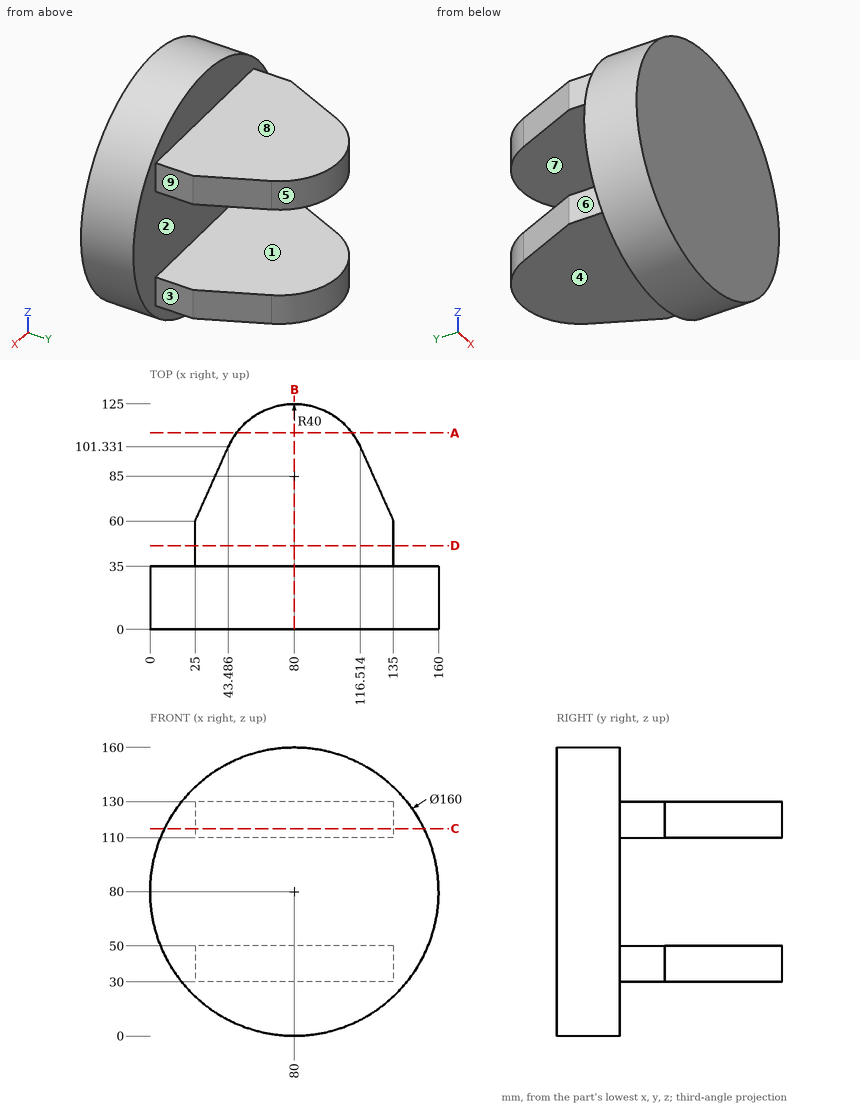
Geometry: see drawing. Coordinates: mm, zero at the bounding-box minimum. A direction names the side the tool comes from. Give positions to 0.01 mm unless a question says otherwise; leave off trailing zeros. Loops run counter-clockwise (first coordinate to the right, second up) from the corner with the lowest first, then second, coordinate; pieces in that order, holes last. Notation, with made-up numbers: (-28.75, -34.75) -> (-3.75, -34.75) arc R13 ccw to (-3.75, -27.75) -> close; hole circle Ø3 at (38, -24.5). An arc over 180 degrees is marked (long way). Answer as a JSON object with one key per item and string values. Group by question number.
Item 1: Cut plane D-D, the plane y = 46.5. Return the cut outline in (x, z), and give its area (3 significant figures).
Item 2: Cut plane C-C, the plane z = 115. Return the cut outline in (x, y).
Item 3: Cut plane A-A, the plane y = 109. Return the cut outline in (x, z), and give its area (3 significant figures).
Item 4: Pin query (flat end, axial travel): P1, Ø4, axis at y = 29, z = 122, coming from the -X side; P2, Ø6, axis at y = 48.5, z = 123, coming from the +X side; P3, Ø8, axis at x = 97.5, z = 84.5, coming from the +Y side. Return the tip coordinate at first contact, or that it passes through.
Item 5: Pull-direction query (Z, two-part tool) for the marked faces 1, 2, 3 and 4; classes: released by +Z, released by -Z, zero draft, split by the parting line, or undercut.
Item 6: Cut plane B-B, the plane x = 80. Return the cut outline in (y, z).
Item 7: Line query: probe 1 along Z at (x, y) = (68, 55); probe 2 along Y at (x, z) = (8, 77); probe 3 along X at (y, z) = (52.5, 115.5). Output: solid intervals per line, ascending.
Item 8: Reachability of the marked faces 5, 6, 7, 8 and 9 from +Z, -Z, +X, -X, +Y, -Y: full face, straight path, thin tool, end or side. Return the list, or none.
Checks:
{
 "1": {"outline": "(25, 30) -> (135, 30) -> (135, 50) -> (25, 50) -> close; (25, 110) -> (135, 110) -> (135, 130) -> (25, 130) -> close", "area": "4,400 mm²"},
 "2": {"outline": "(8.06, 0) -> (151.94, 0) -> (151.94, 35) -> (135, 35) -> (135, 60) -> (116.51, 101.33) arc R40 ccw to (43.49, 101.33) -> (25, 60) -> (25, 35) -> (8.06, 35) -> close"},
 "3": {"outline": "(48, 30) -> (112, 30) -> (112, 50) -> (48, 50) -> close; (48, 110) -> (112, 110) -> (112, 130) -> (48, 130) -> close", "area": "2,560 mm²"},
 "4": {"P1": "stops at x = 10.72", "P2": "stops at x = 135", "P3": "stops at y = 35"},
 "5": {"face 1": "undercut", "face 2": "undercut", "face 3": "zero draft", "face 4": "released by -Z"},
 "6": {"outline": "(0, 0) -> (35, 0) -> (35, 30) -> (125, 30) -> (125, 50) -> (35, 50) -> (35, 110) -> (125, 110) -> (125, 130) -> (35, 130) -> (35, 160) -> (0, 160) -> close"},
 "7": {"probe 1": "z = 30 to 50, 110 to 130", "probe 2": "y = 0 to 35", "probe 3": "x = 25 to 135"},
 "8": {"face 5": "+Z, -Z, +Y", "face 6": "+Z, -Z, -X, +Y", "face 7": "+X, -X, +Y", "face 8": "+Z, +X, -X, +Y", "face 9": "+Z, -Z, +X, +Y"}
}
